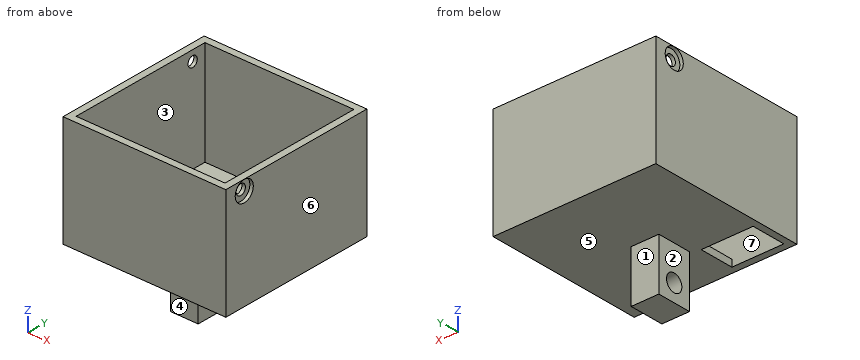
from build123d import *

# Parameters (mm, degrees)
SKETCH1_W         = 47
SKETCH1_H         = 46
SKETCH1_W_2       = 43
SKETCH1_H_2       = 42
WALLS_DEPTH       = 30
SKETCH1_2_W       = 47
SKETCH1_2_H       = 46
SKETCH1_2_W_2     = 43
SKETCH1_2_H_2     = 42
BACK_DEPTH        = 2
SKETCH2_W         = 15
SKETCH2_H         = 10
CABLE_DEPTH       = 2
SKETCH3_R         = 1.5
SETSCREW1_DEPTH   = 2
SKETCH3_6_R       = 2.95
SKETCH3_6_R_2     = 1.5
SETSCREW2_DEPTH   = 1
SETSCREW3_START   = -47
SKETCH3_7_R       = 2.95
SKETCH3_7_R_2     = 1.5
SETSCREW3_DEPTH   = 1
SETSCREW4_START   = -47
SKETCH3_8_R       = 1.5
SETSCREW4_DEPTH   = 2
SKETCH4_W         = 8
SKETCH4_H         = 10
MOUNT_JOINT_DEPTH = 15
SKETCH6_R         = 2.5
JOINT_DEPTH       = 10


with BuildPart() as part:
    # Sketch1 → Walls (new body)
    with BuildSketch(Plane.XY):
        with Locations((-18.175400489, 39.722790127)):
            Rectangle(SKETCH1_W, SKETCH1_H)
        with Locations((-18.175400489, 39.722790127)):
            Rectangle(SKETCH1_W_2, SKETCH1_H_2, mode=Mode.SUBTRACT)
    extrude(amount=WALLS_DEPTH)

    # Sketch1<2> → Back (add)
    # profile 1 of 2: a face of its own
    with BuildSketch(Plane.XY):
        with Locations((-18.175400489, 39.722790127)):
            Rectangle(SKETCH1_2_W, SKETCH1_2_H)
        with Locations((-18.175400489, 39.722790127)):
            Rectangle(SKETCH1_2_W_2, SKETCH1_2_H_2, mode=Mode.SUBTRACT)
    # profile 2 of 2: a face of its own
    with BuildSketch(Plane.XY):
        with Locations((-18.175400489, 39.722790127)):
            Rectangle(SKETCH1_2_W_2, SKETCH1_2_H_2)
    extrude(amount=-BACK_DEPTH)

    # Sketch2 → Cable (cut)
    with BuildSketch(Plane(origin=(0, 0, -2), x_dir=(-1, 0, 0), z_dir=(0, 0, -1))):
        with Locations((32.175400489, 23.722790127)):
            Rectangle(SKETCH2_W, SKETCH2_H)
    extrude(amount=-CABLE_DEPTH, mode=Mode.SUBTRACT)

    # Sketch3 → SetScrew1 (cut)
    with BuildSketch(Plane.ZY.offset(41.675400489)):
        with Locations(Location((27, 56.712532563, 0), (0, 0, 270))):
            Circle(SKETCH3_R)
    extrude(amount=-SETSCREW1_DEPTH, mode=Mode.SUBTRACT)

    # Sketch3<6> → SetScrew2 (cut)
    with BuildSketch(Plane.ZY.offset(41.675400489)):
        with Locations(Location((27, 56.712532563, 0), (0, 0, 270))):
            Circle(SKETCH3_6_R)
        with Locations(Location((27, 56.712532563, 0), (0, 0, 270))):
            Circle(SKETCH3_6_R_2, mode=Mode.SUBTRACT)
    extrude(amount=-SETSCREW2_DEPTH, mode=Mode.SUBTRACT)

    # Sketch3<7> → SetScrew3 (cut)
    with BuildSketch(Plane.ZY.offset(41.675400489).offset(SETSCREW3_START)):
        with Locations(Location((27, 22.733047692, 0), (0, 0, 270))):
            Circle(SKETCH3_7_R)
        with Locations(Location((27, 22.733047692, 0), (0, 0, 270))):
            Circle(SKETCH3_7_R_2, mode=Mode.SUBTRACT)
    extrude(amount=SETSCREW3_DEPTH, mode=Mode.SUBTRACT)

    # Sketch3<8> → SetScrew4 (cut)
    with BuildSketch(Plane.ZY.offset(41.675400489).offset(SETSCREW4_START)):
        with Locations(Location((27, 22.733047692, 0), (0, 0, 270))):
            Circle(SKETCH3_8_R)
    extrude(amount=SETSCREW4_DEPTH, mode=Mode.SUBTRACT)

    # Sketch4 → Mount Joint (add)
    with BuildSketch(Plane(origin=(0, 0, -2), x_dir=(-1, 0, 0), z_dir=(0, 0, -1))):
        with Locations((18.175400489, 34.722790127)):
            Rectangle(SKETCH4_W, SKETCH4_H)
    extrude(amount=MOUNT_JOINT_DEPTH)

    # Sketch6 → Joint (cut)
    with BuildSketch(Plane.ZY.offset(22.175400489)):
        with Locations((-12, 34.722790127)):
            Circle(SKETCH6_R)
    extrude(amount=-JOINT_DEPTH, mode=Mode.SUBTRACT)


solid = part.part
Can you work these out from the model? Positions are in its coordinate system, mm. Face numbers are marked on the shaded views. A direction names the side the tool comes from. Give positions to 0.01 mm unless a question says otherwise; leave off trailing zeros. Loops run counter-clockwise (first coordinate to the right, second up) from the corner with the lowest first, then second, coordinate; pieces in that order, holes last. Notation, with made-up numbers: (37.25, 5.25) -> (55.25, 5.25) arc R20 cw to (55.25, 18.25) -> close; hole circle Ø3 at (60.25, 33.5). An arc over 180 degrees is marked (long way). Return JSON: item names as keys, results as strings.
Q1. I want a section at B-B, the plane x = -38. List the corners of the cut face in (y, z) for me.
Checks:
{"outline": "(16.72, -2) -> (18.72, -2) -> (18.72, 30) -> (16.72, 30) -> close; (28.72, -2) -> (62.72, -2) -> (62.72, 30) -> (60.72, 30) -> (60.72, 0) -> (28.72, 0) -> close"}
Q2. I need wall thicknesses on probe 1 along X at (y, z) = (28, 23); probe 2 along Y at (x, z) = (-6, 15.5); probe 3 along Z at (x, y) = (3, 55). Which ranges of each line are inside material? Lowest first, please.
Checks:
{"probe 1": "x = -41.68 to -39.68, 3.32 to 5.32", "probe 2": "y = 16.72 to 18.72, 60.72 to 62.72", "probe 3": "z = -2 to 0"}
Q3. We'd pull the mould along X, two halves only. Please class the marked faces 5, 6 and 7: released by +X, released by -X, zero draft, split by the parting line, or undercut.
Checks:
{"face 5": "zero draft", "face 6": "released by +X", "face 7": "undercut"}
Q4. For pin 1 Ø5 at (y, z) = (22.73, 27) entering from +X; pin 2 Ø2 at (x, y) = (-7.5, 52) entering from +Z; pin 3 Ø9 at (x, z) = (-18.5, -10) entering from +Y; pin 4 Ø14 at (x, y) = (-8.5, 34) entering from -Z, each with a flat end and sliding along its axis, tell me the tip position at first contact or that it passes through.
Checks:
{"pin 1": "stops at x = 4.32", "pin 2": "stops at z = 0", "pin 3": "stops at y = 39.72", "pin 4": "stops at z = -17"}
Q5. I want a section at A-A, the plane z = -12. List the corners of the cut face in (x, y) for me, then the cut area to 3 significant figures.
Checks:
{"outline": "(-22.18, 29.72) -> (-14.18, 29.72) -> (-14.18, 32.22) -> (-22.18, 32.22) -> close; (-22.18, 37.22) -> (-14.18, 37.22) -> (-14.18, 39.72) -> (-22.18, 39.72) -> close", "area": "40.0 mm2"}
Q6. I want a section at D-D, the plane z = 17. List the corners of the cut face in (x, y) for me, then the cut area to 3 significant figures.
Checks:
{"outline": "(-41.68, 16.72) -> (5.32, 16.72) -> (5.32, 62.72) -> (-41.68, 62.72) -> close; hole (-39.68, 18.72) -> (3.32, 18.72) -> (3.32, 60.72) -> (-39.68, 60.72) -> close", "area": "356 mm2"}
Q7. I want a section at C-C, the plane x = -13. List the corners of the cut face in (y, z) for me, then the cut area to 3 significant figures.
Checks:
{"outline": "(16.72, -2) -> (62.72, -2) -> (62.72, 30) -> (60.72, 30) -> (60.72, 0) -> (18.72, 0) -> (18.72, 30) -> (16.72, 30) -> close", "area": "212 mm2"}
Q8. On a 3-axis mill with a long thin cutter (end or side, diameter ignored), from which of +Z, -Z, +X, -X, +Y, -Y can I reach the whole of each face in a straight line? I mean the marked faces 1, 2, 3 and 4. Say none if no direction works.
Checks:
{"face 1": "-Z, +X, -X, +Y", "face 2": "-Z, -X, +Y, -Y", "face 3": "+Z", "face 4": "-Z, +X, -X, -Y"}
